Part model, mm, in its own coordinate system. Face numbers are marked on the shaded views. A direction names the side the tool comes from. Round coordinates to 2 decimals unless told otherwise and drop trailing zeros. Loops run counter-clockwise (first coordinate to the right, second up) from the corner with the lowest first, then second, coordinate; pieces in that order, holes last.
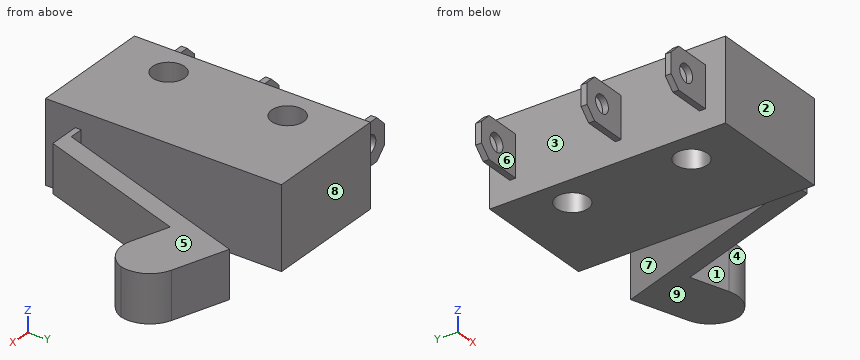
from build123d import *

# Parameters (mm, degrees)
F0_W         = 10.4
F0_H         = 19.9
F1_DEPTH     = 6.9
F2_R         = 1.35
F3_DEPTH     = 6.9
F4_W         = 0.5
F4_H         = 1.746198668
F5_DEPTH     = 4
F7_DEPTH     = 16.5
F8_W         = 0.5
F8_H         = 2
F9_DEPTH     = 1.15
F11_DEPTH    = 4
F12_W        = 1.55500961
F12_H        = 4
F13_DEPTH    = 18.65
F14_W        = 4.8
F14_H        = 4
F15_DEPTH    = 5.85
F16_T1_DEPTH = 16.7


# Not quite as in the source:
# - a fillet or chamfer that OpenCascade refuses, or shapes differently, is made with other operations: its cross-section is extruded or revolved along the edge and cut away or added


with BuildPart() as f1:
    # F0 (on Top) → F1 (new body)
    with BuildSketch(Plane.XY):
        Rectangle(F0_W, F0_H)
    extrude(amount=F1_DEPTH)

    # F2 (on face) → F3 (cut, through all)
    with BuildSketch(Plane.XY.offset(6.9)):
        with Locations((-2.6, 4.85)):
            Circle(F2_R)
        with Locations((-2.6, -5.2)):
            Circle(F2_R)
    extrude(amount=-F3_DEPTH, mode=Mode.SUBTRACT)

    # F4 (on face) → F5 (join)
    with BuildSketch(Plane(origin=(-5.2, 0, 0), x_dir=(0, -1, 0), z_dir=(-1, 0, 0))):
        with Locations((-8, 2.576900666)):
            Rectangle(F4_W, F4_H)
        with Locations((8, 4.323099334)):
            Rectangle(F4_W, F4_H)
        with Locations((8, 2.576900666)):
            Rectangle(F4_W, F4_H)
        with Locations((0.9, 4.323099334)):
            Rectangle(F4_W, F4_H)
        with Locations((0.9, 2.576900666)):
            Rectangle(F4_W, F4_H)
        with Locations((-8, 4.323099334)):
            Rectangle(F4_W, F4_H)
    extrude(amount=F5_DEPTH)

    # F6 (on face) → F7 (cut, through all)
    with BuildSketch(Plane(origin=(0, 8.25, 0), x_dir=(-1, 0, 0), z_dir=(0, 1, 0))):
        with BuildLine():
            Line((6.7, 3.45), (8.2, 3.45))
            ThreePointArc((8.2, 3.45), (7.45, 4.2), (6.7, 3.45))
        make_face()
        with BuildLine():
            ThreePointArc((6.7, 3.45), (7.45, 2.7), (8.2, 3.45))
            Line((8.2, 3.45), (6.7, 3.45))
        make_face()
        Polygon((9.2, 5.196198668), (8.3137443289, 5.196198668), (9.2, 4.3099429969), align=None)
        Polygon((9.2, 1.703801332), (9.2, 2.5900570031), (8.3137443289, 1.703801332), align=None)
    extrude(amount=-F7_DEPTH, mode=Mode.SUBTRACT)

    # F8 (on face) → F9 (join)
    with BuildSketch(Plane.YZ.offset(5.2)):
        with Locations((-7.2, 2.45)):
            Rectangle(F8_W, F8_H)
        with Locations((-7.2, 4.45)):
            Rectangle(F8_W, F8_H)
    extrude(amount=F9_DEPTH)

    # F10 (on face) → F11 (join, through all)
    with BuildSketch(Plane(origin=(0, 0, 1.45), x_dir=(1, 0, 0), z_dir=(0, 0, -1))):
        Polygon((6.35, 7.45), (6.35, 6.95), (7.8224316239, 7.45), align=None)
    extrude(amount=-F11_DEPTH)

    # F12 (on face) → F13 (join)
    with BuildSketch(Plane(origin=(-1.4595201755, -4.2980873242, 0), x_dir=(-0.946895514, 0.3215414212, 0), z_dir=(0.3215414212, 0.946895514, 0))):
        with Locations((-9.0250041964, 3.45)):
            Rectangle(F12_W, F12_H)
    extrude(amount=F13_DEPTH)

    # F14 (on face) → F15 (join)
    with BuildSketch(Plane(origin=(9.2819517994, -3.1519126758, 0), x_dir=(0.3215414212, 0.946895514, 0), z_dir=(0.946895514, -0.3215414212, 0))):
        with Locations((11.7108642024, 3.45)):
            Rectangle(F14_W, F14_H)
    extrude(amount=F15_DEPTH)

    # F16: fillet of radius 2.54 on 2 edges, made by hand

    # F16_s2 → F16_t1 (cut)
    with BuildSketch(Plane.XY.offset(-4.9)):
        with BuildLine():
            ThreePointArc((16.953403281, 9.145299232), (18.4148657814, 7.8633526103), (18.5418026766, 5.9234694165))
            Line((18.5418026766, 5.9234694165), (19.3585178865, 8.3285840221))
            Line((19.3585178865, 8.3285840221), (16.953403281, 9.145299232))
        make_face()
        with BuildLine():
            ThreePointArc((18.6318342746, 6.1886001604), (17.3498876529, 4.72713766), (15.4100044591, 4.6002007647))
            Line((15.4100044591, 4.6002007647), (17.8151190647, 3.7834855549))
            Line((17.8151190647, 3.7834855549), (18.6318342746, 6.1886001604))
        make_face()
    extrude(amount=F16_T1_DEPTH, mode=Mode.SUBTRACT)


solid = f1.part
1) Drop flat-ended pins along their axis: pin 1 Ø4 at (x, y) = (10.5, -5.5) entering from +Z; pin 2 Ø2 at (x, y) = (-2.6, 4.85) entering from +Z; pin 3 Ø2 at (y, z) = (5.5, 2.5) entering from +X; pin 4 Ø11 at (x, y) = (15, 5.5) entering from -Z. Give the stop position or say it passes through.
Values:
pin 1: stops at z = 5.45
pin 2: passes through
pin 3: stops at x = 18.67
pin 4: stops at z = 1.45
2) Slice it at A-A, the plane x = -7.45. Give the cut face in (y, z).
Values:
outline: (-8.25, 1.7) - (-7.75, 1.7) - (-7.75, 2.7) - (-8.25, 2.7) - close; (-8.25, 4.2) - (-7.75, 4.2) - (-7.75, 5.2) - (-8.25, 5.2) - close; (-1.15, 1.7) - (-0.65, 1.7) - (-0.65, 2.7) - (-1.15, 2.7) - close; (-1.15, 4.2) - (-0.65, 4.2) - (-0.65, 5.2) - (-1.15, 5.2) - close; (7.75, 1.7) - (8.25, 1.7) - (8.25, 2.7) - (7.75, 2.7) - close; (7.75, 4.2) - (8.25, 4.2) - (8.25, 5.2) - (7.75, 5.2) - close
3) Mould opens along X. For the marked faces 1, 2, 3 and 4 say: released by +X, released by -X, zero draft, split by the parting line, or undercut.
Values:
face 1: undercut
face 2: zero draft
face 3: released by -X
face 4: undercut
4) Slice it at D-D, the plane y = -3. Give the cut face in (x, z), then the cut area to 3 significant figures.
Values:
outline: (-5.2, 0) - (5.2, 0) - (5.2, 6.9) - (-5.2, 6.9) - close; (7.69, 1.45) - (9.33, 1.45) - (9.33, 5.45) - (7.69, 5.45) - close
area: 78.3 mm2
5) Slice it at C-C, the plane x = -2.6. Give the cut face in (y, z), then the cut area to 3 significant figures.
Values:
outline: (-9.95, 0) - (-6.55, 0) - (-6.55, 6.9) - (-9.95, 6.9) - close; (-3.85, 0) - (3.5, 0) - (3.5, 6.9) - (-3.85, 6.9) - close; (6.2, 0) - (9.95, 0) - (9.95, 6.9) - (6.2, 6.9) - close
area: 100 mm2
6) Slice it at B-B, the plane z = 6.5. Give the cut face in (x, y).
Values:
outline: (-5.2, -9.95) - (5.2, -9.95) - (5.2, 9.95) - (-5.2, 9.95) - close; hole circle Ø2.7 at (-2.6, -5.2); hole circle Ø2.7 at (-2.6, 4.85)
7) Wall check: line 1 along Y through (x, z) = (-2.6, 2); line 2 along Z through (x, y) = (-7.45, 8.1); line 3 along X through (y, z) = (-1, 3.45). Give the ranges that are in metal, low to high.
Values:
line 1: y = -9.95 to -6.55, -3.85 to 3.5, 6.2 to 9.95
line 2: z = 1.7 to 2.7, 4.2 to 5.2
line 3: x = -9.2 to -8.2, -6.7 to 5.2, 8.37 to 10.01
8) Tool access for the marked faces 5, 6, 7, 8 and 9: list every direction of +Z, -Z, +X, -X, +Y, -Y with a clear straight run to the whole face (end or side of a thin tool).
Values:
face 5: +Z, +X, +Y, -Y
face 6: +Z, -Z, -X
face 7: +Z, -Z, +Y
face 8: +Z, -Z, -X, +Y
face 9: -Z, +X, +Y, -Y
